Could you check a few things on this model? Use its own coordinates, in mm. Round coordinates to 2 decimals unless told otherwise and drop trailing zeros. Order: outer loops, then holes, each group sorted by start corner. A loop starts at its lowest first (then second) coordinate and runs counter-clockwise, first axis right, second up. Notation, with made-up numbers: (1.5, 39) -> (16.5, 39) arc R11 ccw to (16.5, 60) -> close; hole circle Ø5 at (-12, 84.25). An arc over 180 degrees is marked (long way). Put each result on its own line as item: value. Start each with the question number.
from build123d import *

# Parameters (mm, degrees)
SKETCH1_R           = 35
BOSS_EXTRUDE1_DEPTH = 5
SKETCH2_R           = 3.1
CUT_EXTRUDE1_DEPTH  = 50.749371855
SKETCH3_W           = 12.74
SKETCH3_H           = 10.8
CUT_EXTRUDE2_DEPTH  = 5
CIRPATTERN1_COUNT   = 4
SKETCH4_W           = 12.74
SKETCH4_H           = 5
CUT_EXTRUDE3_DEPTH  = 75.344872049
CIRPATTERN2_COUNT   = 4
CUT_EXTRUDE4_DEPTH  = 2


with BuildPart() as part:
    # Sketch1 → Boss-Extrude1 (new body)
    with BuildSketch(Plane(origin=(0, 0, 0), x_dir=(1, 0, 0), z_dir=(0, 1, 0))):
        with Locations(Location((0, 0, 0), (0, 0, 270))):
            Circle(SKETCH1_R)
    extrude(amount=BOSS_EXTRUDE1_DEPTH)

    # Sketch2 → Cut-Extrude1 (cut, through all)
    with BuildSketch(Plane(origin=(0, 5, 0), x_dir=(1, 0, 0), z_dir=(0, 1, 0))):
        with Locations(Location((-17.67766953, 17.67766953, 0), (0, 0, 270))):
            Circle(SKETCH2_R)
        with Locations(Location((17.67766953, 17.67766953, 0), (0, 0, 270))):
            Circle(SKETCH2_R)
        with Locations(Location((17.67766953, -17.67766953, 0), (0, 0, 270))):
            Circle(SKETCH2_R)
        with Locations(Location((-17.67766953, -17.67766953, 0), (0, 0, 270))):
            Circle(SKETCH2_R)
    extrude(amount=-CUT_EXTRUDE1_DEPTH, mode=Mode.SUBTRACT)

    # Sketch3 → Cut-Extrude2 (cut)
    with BuildSketch(Plane(origin=(0, 5, 0), x_dir=(1, 0, 0), z_dir=(0, 1, 0))):
        with Locations((0, 25)):
            Rectangle(SKETCH3_W, SKETCH3_H)
    cut_extrude2 = extrude(amount=-CUT_EXTRUDE2_DEPTH, mode=Mode.SUBTRACT)

    # CirPattern1: Cut-Extrude2 ×4 about axis
    cirpattern1_axis = Axis((0, 0, 0), (0, 1, 0))
    for i in range(1, CIRPATTERN1_COUNT):
        add(cut_extrude2.rotate(cirpattern1_axis, i * 360 / CIRPATTERN1_COUNT), mode=Mode.SUBTRACT)

    # Sketch4 → Cut-Extrude3 (cut, through all)
    with BuildSketch(Plane.XY.offset(-30.4)):
        with Locations((0, 2.5)):
            Rectangle(SKETCH4_W, SKETCH4_H)
    cut_extrude3 = extrude(amount=-CUT_EXTRUDE3_DEPTH, mode=Mode.SUBTRACT)

    # CirPattern2: Cut-Extrude3 ×4 about axis
    cirpattern2_axis = Axis((0, 5, 0), (0, 1, 0))
    for i in range(1, CIRPATTERN2_COUNT):
        add(cut_extrude3.rotate(cirpattern2_axis, i * 360 / CIRPATTERN2_COUNT), mode=Mode.SUBTRACT)

    # Sketch5 → Cut-Extrude4 (cut)
    with BuildSketch(Plane.XZ):
        with BuildLine():
            Line((-19.6, -6.37), (-34.415448566, -6.37))
            ThreePointArc((-34.415448566, -6.37), (-24.748737342, -24.748737342), (-6.37, -34.415448566))
            Line((-6.37, -34.415448566), (-6.37, -19.6))
            Line((-6.37, -19.6), (6.37, -19.6))
            Line((6.37, -19.6), (6.37, -34.415448566))
            ThreePointArc((6.37, -34.415448566), (24.748737342, -24.748737342), (34.415448566, -6.37))
            Line((34.415448566, -6.37), (19.6, -6.37))
            Line((19.6, -6.37), (19.6, 6.37))
            Line((19.6, 6.37), (34.415448566, 6.37))
            ThreePointArc((34.415448566, 6.37), (24.748737342, 24.748737342), (6.37, 34.415448566))
            Line((6.37, 34.415448566), (6.37, 19.6))
            Line((6.37, 19.6), (-6.37, 19.6))
            Line((-6.37, 19.6), (-6.37, 34.415448566))
            ThreePointArc((-6.37, 34.415448566), (-24.748737342, 24.748737342), (-34.415448566, 6.37))
            Line((-34.415448566, 6.37), (-19.6, 6.37))
            Line((-19.6, 6.37), (-19.6, -6.37))
        make_face()
    extrude(amount=-CUT_EXTRUDE4_DEPTH, mode=Mode.SUBTRACT)


solid = part.part
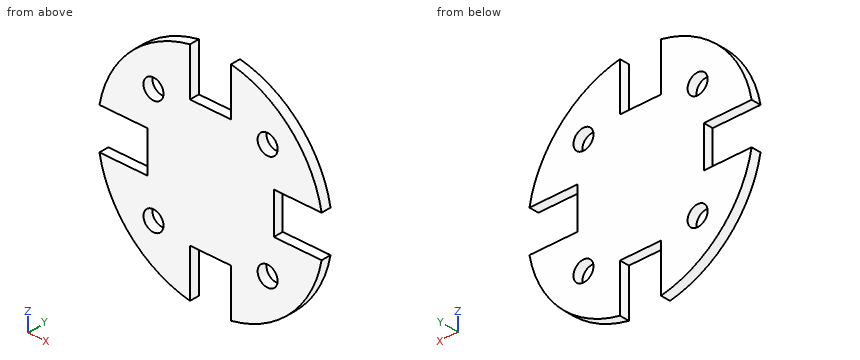
1. I need wall thicknesses on L1, parallel to Z at x = 19.5, y = 4.4; L2, parallel to Z at x = -20.5, y = 3.55; L3, parallel to Z at x = 24.5, y = 2.4 (3 decimals). Which ranges of each line are inside material? Lowest first, please.
2. If we section it at C-C, the plane y = 3.2: Please give me the cut outline in (x, z).
3. If we section it at B-B, the plane z = 16.5: Please give me the cut outline in (x, y).
4. For pin 1 Ø3.5 at (x, z) = (17.68, 17.68) entering from +Y; pin 2 Ø10 at (x, z) = (16.5, 15.5) entering from +Y; pin 3 Ø1.5 at (x, y) = (30, 3) entering from +Z; pin 4 Ø0.9 at (y, z) = (4, -2) entering from -X, each with a flat end and sliding along its axis, tell me the tip position at first contact or that it passes through.
5. If we section it at A-A, the plane x = 28: Please give me the cut outline in (y, z).
6. If we section it at D-D, the plane x = -15.5: Please give me the cut outline in (y, z).
Results below:
1. L1: -29.06 to -20.19, -15.17 to 15.17, 20.19 to 29.06
1. L2: -28.37 to -18.96, -16.4 to -6.37, 6.37 to 16.4, 18.96 to 28.37
1. L3: -24.995 to -6.37, 6.37 to 24.995
2. outline: (-34.42, -6.37) arc R35 ccw to (-6.37, -34.42) -> (-6.37, -19.6) -> (6.37, -19.6) -> (6.37, -34.42) arc R35 ccw to (34.42, -6.37) -> (19.6, -6.37) -> (19.6, 6.37) -> (34.42, 6.37) arc R35 ccw to (6.37, 34.42) -> (6.37, 19.6) -> (-6.37, 19.6) -> (-6.37, 34.42) arc R35 ccw to (-34.42, 6.37) -> (-19.6, 6.37) -> (-19.6, -6.37) -> close; hole circle Ø6.2 at (-17.68, -17.68); hole circle Ø6.2 at (-17.68, 17.68); hole circle Ø6.2 at (17.68, -17.68); hole circle Ø6.2 at (17.68, 17.68)
3. outline: (-30.87, 2) -> (-20.55, 2) -> (-20.55, 5) -> (-30.87, 5) -> close; (-14.81, 2) -> (14.81, 2) -> (14.81, 5) -> (-14.81, 5) -> close; (20.55, 2) -> (30.87, 2) -> (30.87, 5) -> (20.55, 5) -> close
4. pin 1: through
4. pin 2: y = 5
4. pin 3: z = 19.22
4. pin 4: x = -19.6
5. outline: (2, -21) -> (5, -21) -> (5, -6.37) -> (2, -6.37) -> close; (2, 6.37) -> (5, 6.37) -> (5, 21) -> (2, 21) -> close
6. outline: (2, -31.38) -> (5, -31.38) -> (5, -19.88) -> (2, -19.88) -> close; (2, -15.47) -> (5, -15.47) -> (5, 15.47) -> (2, 15.47) -> close; (2, 19.88) -> (5, 19.88) -> (5, 31.38) -> (2, 31.38) -> close
